Autodesk Inventor part; units mm, degrees
ref_plane "YZ Plane" through (0, 0, 0) normal (1, 0, 0) x (0, 1, 0)
ref_plane "XZ Plane" through (0, 0, 0) normal (0, 1, 0) x (-1, 0, 0)
ref_plane "XY Plane" through (0, 0, 0) normal (0, 0, 1) x (1, 0, 0)
sketch "スケッチ1" plane through (0, 0, 0) normal (0, 1, 0) x (-1, 0, 0)
  line L0 (0, 0) -> (-5, 0)
  line L1 (-5, 0) -> (-5, -5)
  line L2 (-5, -5) -> (0, -5)
  line L3 (0, -5) -> (0, 0)
  dimension "d0" = 5
  dimension "d1" = 5
extrude "押し出し1" add sketch "スケッチ1" along normal blind 7.5
sketch "スケッチ2" plane through (0, 0, 0) normal (0, 0, 1) x (1, 0, 0)
  line L0 (0, 0) -> (5, 0)
  line L1 (0, 0) -> (0, 7.5)
  point P0 (2.5, 2.5)
  dimension "d11" = 2.5
  dimension "d12" = 2.5
hole "穴1" at (2.5, 2.5, 0) direction (0, 0, -1) diameter 3.1 end through all
sketch "スケッチ3" plane through (0, 0, 0) normal (0, 0, 1) x (1, 0, 0)
  line L0 (1, 7.5) -> (4, 7.5)
  line L1 (4, 7.5) -> (4, 5)
  line L2 (4, 5) -> (1, 5)
  line L3 (1, 5) -> (1, 7.5)
  line L4 (1, 7.5) -> (4, 5) construction
  line L5 (4, 7.5) -> (1, 5) construction
  line L6 (0, 0) -> (0, 7.5)
  line L7 (0, 7.5) -> (5, 7.5)
  point P0 (2.5, 6.25)
  dimension "d13" = 3
  dimension "d14" = 2.5
  dimension "d15" = 2.5
  dimension "d16" = 0
extrude "押し出し2" cut sketch "スケッチ3" against normal through all
fillet "フィレット1" radius 2 2 edges at (5, 0, -2.5) (0, 0, -2.5)
fillet "フィレット2" radius 0.5 4 edges at (1, 6.25, 0) (4, 6.25, 0) (1, 6.25, -5) (4, 6.25, -5)
properties part number "gomu_guide2.8"
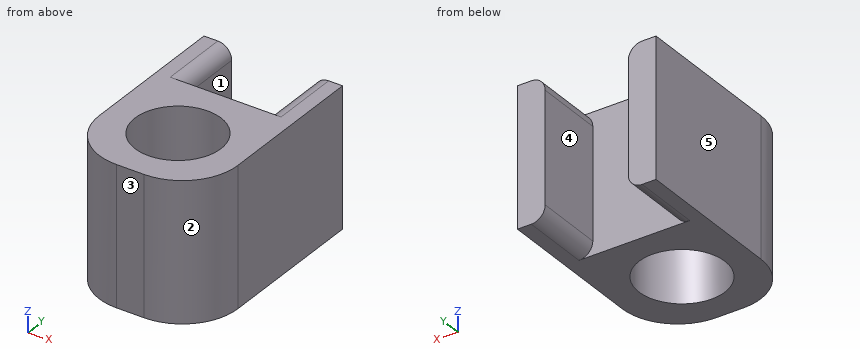
Design review of the part built by this model. Coordinates are the model's own, in mm. Face numbers are marked on the shaded views. A direction names the side the tool comes from. Round coordinates to 2 decimals unless told otherwise and drop trailing zeros. Write each loop counter-clockwise with the first axis right and the second up, starting at its lowest first coordinate (ties: lowest second). Pieces come first, ordered by that corner, then holes. Notation, with made-up numbers: M 61,34.5 L 80,34.5 A22 ccw 80,61.5 Z; hole C 74,-14.5 d3. An arc over 180 degrees is marked long. One line per item, written item: value. Start each with the question number.
1. To check wall thickness, follow probe 1 along X at (y, z) = (2.5, -2.45); probe 2 along X at (y, z) = (3.25, -3). State the ranges of each line that lie inside material, in increasing order. Write a range as from..to.
2. Take a section at B-B on z = -3.5. State the section outline as (x, y) points, then the cut area to 3 significant figures.
3. Draft analysis for pull direction X (two halves, no side actions). For the marked faces 1, 2 and 3, state which applies: pulls with the +X half, pulls with the -X half, needs draft (parallel to the pull), parting line crosses it, or undercut.
4. Clearance check with a flat-ended pin moving along its axis: P1, Ø1.5, axis at x = 2, z = -0.5, coming from the +Y side. State where the tip first meets the part, or that it passes through.
5. Take a section at D-D on x = 4.6. State the section outline as (y, z) points, then the cut area to 3 significant figures.
6. For the marked faces 4 and 5, list the 3-axis set-ups (+Z, -Z, +X, -X, +Y, -Y) from which the entire face can be reached by the end or side of a thin tool; tool diameter is ignored.
7. Take a section at A-A on x = 2.5. State the section outline as (y, z) points.
Computed:
1. probe 1: x = 0..0.95, 4.05..5
1. probe 2: x = 0..1.14, 3.86..5
2. outline: M 0,2 A2 ccw 2,0 L 3,0 A2 ccw 5,2 L 5,7.5 L 4,7.5 L 4,5 L 1,5 L 1,7.5 L 0,7.5 Z; hole C 2.5,2.5 d3.1
2. area: 20.7 mm²
3. face 1: undercut
3. face 2: pulls with the +X half
3. face 3: needs draft
4. P1: stops at y = 5
5. outline: M 0.8,-5 L 7.5,-5 L 7.5,0 L 0.8,0 Z
5. area: 33.5 mm²
6. face 4: +Z, -Z, +Y
6. face 5: +Z, -Z, -X, +Y, -Y
7. outline: M 0,-5 L 0.95,-5 L 0.95,0 L 0,0 Z; M 4.05,-5 L 5,-5 L 5,0 L 4.05,0 Z
